Input: part model. Units: mm. Frame: model coordinates. Round coordinates to 2 decimals unless told otherwise and drop trailing zeros. Loops run counter-clockwise (first coordinate to the right, second up) from the corner with the lowest first, then second, coordinate; pieces in that order, holes last. Notation, with made-up numbers: M -32,14 L 26,14 A17 ccw 26,24 Z; hole C -31,52.5 d8. An arc over 180 degrees is marked long. Use one line per item in the form item = value. Start each with the question number.
Q1. First-contact query: P1, Ø6, axis at x = -399, z = 16, coming from the -Y side; P2, Ø12, axis at x = -444, z = 3, coming from the -Y side. Flat tips, straight axial feed; report the tip coordinate or a pass-through.
Q2. Section query D-D, the plane y = 112.5. Output: boundary loops of the cut face in (x, z), and give its area (3 significant figures).
Q3. Section query C-C, the plane x = -80. Output: boundary loops of the cut face in (y, z), and give its area (3 significant figures).
Q4. Mould query, pull axis Y, two halves, no side actions, for faces 1 (the flat face through (-542, 309, 0)), 2 (the cylindrical face through (-103.81, 94.25, 9.86)), 3 (the flat face through (-1004, 0, 10)). Classes: pulls with the +Y half, pulls with the -Y half, needs draft (parallel to the pull), parting line crosses it, or undercut.
Q5. Ray query, line 1 along Y through (x, z) = (-80, 10.25); line 2 along Y through (x, z) = (-58.5, 19); line 3 along X through (y, z) = (374.5, 17). Return the intervals inside material, ascending.
Q6. Section query A-A, the plane y = 387.5. Output: boundary loops of the cut face in (x, z).
Q7. Section query B-B, the plane z = 6. Output: boundary loops of the cut face in (x, y), and give its area (3 significant figures).
```python
from build123d import *

# Parameters (mm, degrees)
IZIM1_R                     = 30
Y_KSEKLIK_EKSTR_ZYON1_DEPTH = 20
KES_EKSTR_ZYON1_DEPTH       = 20


with BuildPart() as part:
    # Çizim1 → Yükseklik-Ekstrüzyon1 (new body)
    with BuildSketch(Plane.XY):
        with BuildLine():
            Line((-30, 0), (-1070, 0))
            ThreePointArc((-1070, 0), (-1091.213203436, 8.786796564), (-1100, 30))
            Line((-1100, 30), (-1100, 470))
            ThreePointArc((-1100, 470), (-1091.213203436, 491.213203436), (-1070, 500))
            Line((-1070, 500), (-30, 500))
            ThreePointArc((-30, 500), (-8.786796564, 491.213203436), (0, 470))
            Line((0, 470), (0, 30))
            ThreePointArc((0, 30), (-8.786796564, 8.786796564), (-30, 0))
        make_face()
        with Locations((-1020, 387.5)):
            Circle(IZIM1_R, mode=Mode.SUBTRACT)
        with Locations((-80, 112.5)):
            Circle(IZIM1_R, mode=Mode.SUBTRACT)
    extrude(amount=Y_KSEKLIK_EKSTR_ZYON1_DEPTH)

    # Çizim2 → Kes-Ekstrüzyon1 (cut)
    with BuildSketch(Plane(origin=(0, 0, 0), x_dir=(-1, 0, 0), z_dir=(0, 0, -1))):
        with BuildLine():
            Line((940, 0), (160, 0))
            ThreePointArc((160, 0), (550, 250), (940, 0))
        make_face()
    extrude(amount=-KES_EKSTR_ZYON1_DEPTH, mode=Mode.SUBTRACT)


solid = part.part
```
Results found:
q1.P1 = 221.42
q1.P2 = 235.13
q2.outline = M -1100,0 L -864.84,0 L -864.84,20 L -1100,20 Z; M -235.16,0 L -110,0 L -110,20 L -235.16,20 Z; M -50,0 L 0,0 L 0,20 L -50,20 Z
q2.area = 8,210 mm²
q3.outline = M 0,0 L 82.5,0 L 82.5,20 L 0,20 Z; M 142.5,0 L 500,0 L 500,20 L 142.5,20 Z
q3.area = 8,800 mm²
q4.face_1 = needs draft
q4.face_2 = undercut
q4.face_3 = pulls with the -Y half
q5.line_1 = 0 to 82.5, 142.5 to 500
q5.line_2 = 0 to 91.58, 133.42 to 500
q5.line_3 = -1100 to -1047.04, -992.96 to 0
q6.outline = M -1100,0 L -1050,0 L -1050,20 L -1100,20 Z; M -990,0 L 0,0 L 0,20 L -990,20 Z
q7.outline = M -1100,30 A30 ccw -1070,0 L -940,0 A429.2 cw -160,0 L -30,0 A30 ccw 0,30 L 0,470 A30 ccw -30,500 L -1070,500 A30 ccw -1100,470 Z; hole C -1020,387.5 d60; hole C -80,112.5 d60
q7.area = 403,000 mm²
